```python
from build123d import *

# Parameters (mm, degrees)
F0_W     = 68.58
F0_H     = 68.58
F1_DEPTH = 50.8
F1_TAPER = 34
F2_SCALE = 0.74


with BuildPart() as f1:
    # F0 (on Top) → F1 (new body)
    with BuildSketch(Plane.XY):
        Rectangle(F0_W, F0_H)
    extrude(amount=F1_DEPTH, taper=F1_TAPER)


with BuildPart() as f1_1:
    # F2: moved
    add(f1.part.scale(F2_SCALE))

    # F3: F1 across plane


with BuildPart() as f1_2:
    add(f1_1.part)
    add(f1_1.part.mirror(Plane.XY))


solid = f1_2.part
```
CAD build for the part. Positions are in the model's coordinates, mm. Give positions to 0.01 mm unless a question says otherwise; leave off trailing zeros. Order: outer loops, then holes, each group sorted by start corner. A loop starts at its lowest first (then second) coordinate and runs counter-clockwise, first axis right, second up. Notation, with made-up numbers: M 8.5,72.5 L 63.5,72.5 A36 cw 63.5,106.5 Z; hole C 86.25,30.5 d1. An arc over 180 degrees is marked long. Put each result on its own line as item: value. Start each with the question number.
(1) Saw through at B-B, the plane x = 20. Write the cut outline in (y, z).
(2) Saw through at A-A, the plane y = -11. Write the cut outline in (x, z), then the cut area to 3 significant figures.
(3) Drill centre lines: line 1 along Z through (x, y) = (-9, -1); line 2 along Z through (x, y) = (-17.5, -14); line 3 along X through (y, z) = (7, 22). Where is each one in solid material? Low to high.
(4) Saw through at D-D, the plane z = 8.5. Write the cut outline in (x, y), then the cut area to 3 significant figures.
(5) Flat gauge pins, fed straight in: pin 1 Ø4 at (y, z) = (-5.5, -6.5) entering from -X; pin 2 Ø10 at (x, z) = (10.5, 15) entering from +Y; pin 3 Ø4 at (x, y) = (20, -15.5) entering from -Z; pin 4 Ø10 at (x, z) = (7.5, 4.5) entering from -Y. Where does each tip first touch, or does it go through?
(6) Mould opens along Z. For faces 1 (the flat face through (-0.36, 15.69, -14.36)), 2 (the flat face through (-15.69, -0.36, 14.36)) say: +Z half, -Z half, draft (parallel to the pull), parting line (faces both ways), or undercut.
(7) Saw through at C-C, the plane z = 28.5. Write the cut outline in (x, y).
Check result:
1. outline: M -25.37,0 L -20,-7.97 L 20,-7.97 L 25.37,0 L 20,7.97 L -20,7.97 Z
2. outline: M -25.37,0 L -11,-21.31 L 11,-21.31 L 25.37,0 L 11,21.31 L -11,21.31 Z
2. area: 1,550 mm2
3. line 1: z = -24.28 to 24.28
3. line 2: z = -11.67 to 11.67
3. line 3: x = -10.54 to 10.54
4. outline: M -19.64,-19.64 L 19.64,-19.64 L 19.64,19.64 L -19.64,19.64 Z
4. area: 1,540 mm2
5. pin 1: stops at x = -22.34
5. pin 2: stops at y = 18.63
5. pin 3: stops at z = -10.93
5. pin 4: stops at y = -25.37
6. face 1: -Z half
6. face 2: +Z half
7. outline: M -6.15,-6.15 L 6.15,-6.15 L 6.15,6.15 L -6.15,6.15 Z
